from build123d import *

# Parameters (mm, degrees)
SKETCH_1_W              = 48
SKETCH_1_H              = 20
EXTRUDE_1_DEPTH         = 30
SKETCH_2_W              = 14
SKETCH_2_H              = 30
CUT_EXTRUDE_1_DEPTH     = 7
EXTRUDE_2_DEPTH         = 48
CUT_EXTRUDE_2_DEPTH     = 14
CUT_EXTRUDE_3_DEPTH     = 14
CUT_EXTRUDE_4_DEPTH     = 65.456478054
SKETCH_13_R             = 4
CUT_EXTRUDE_5_DEPTH     = 53.52066051
SKETCH_14_R             = 4
CUT_EXTRUDE_6_DEPTH     = 53.52066051
FILLET_1_R              = 7
EXTRUDE_3_DEPTH         = 3
EXTRUDE_5_DEPTH         = 1
SKETCH_20_R             = 7.5
CUT_EXTRUDE_8_DEPTH     = 53.520660579
BOSS_EXTRUDE1_DEPTH     = 25
CUT_EXTRUDE1_DEPTH      = 80.244164279
CUT_EXTRUDE1_DEPTH_BACK = 80.244164279


with BuildPart() as part:
    # Эскиз1 → Бобышка-Вытянуть1 (new body)
    with BuildSketch(Plane(origin=(0, 0, 0), x_dir=(1, 0, 0), z_dir=(0, 1, 0))):
        Rectangle(SKETCH_1_W, SKETCH_1_H)
    extrude(amount=EXTRUDE_1_DEPTH)

    # Эскиз2 → Вырез-Вытянуть1 (cut)
    with BuildSketch(Plane.XY.offset(10)):
        with Locations((0, 15)):
            Rectangle(SKETCH_2_W, SKETCH_2_H)
    extrude(amount=-CUT_EXTRUDE_1_DEPTH, mode=Mode.SUBTRACT)

    # Эскиз7 → Бобышка-Вытянуть2 (add)
    with BuildSketch(Plane(origin=(24, 0, 0), x_dir=(0, 0, -1), z_dir=(1, 0, 0))):
        Polygon((10, 0), (27.320508076, -10), (45.810889132, 22.026279442), (32, 30), (10, 30), align=None)
    extrude(amount=-EXTRUDE_2_DEPTH)

    # Эскиз8 → Вырез-Вытянуть2 (cut)
    with BuildSketch(Plane(origin=(24, 0, 0), x_dir=(0, 0, -1), z_dir=(1, 0, 0))):
        Polygon((10, 0), (10, 30), (32, 30), (45.810889132, 22.026279442), (27.320508076, -10), align=None)
    extrude(amount=-CUT_EXTRUDE_2_DEPTH, mode=Mode.SUBTRACT)

    # Эскиз9 → Вырез-Вытянуть3 (cut)
    with BuildSketch(Plane.ZY.offset(24)):
        Polygon((-10, 0), (-10, 30), (-32, 30), (-45.810889132, 22.026279442), (-27.320508076, -10), align=None)
    extrude(amount=-CUT_EXTRUDE_3_DEPTH, mode=Mode.SUBTRACT)

    # Эскиз11 → Вырез-Вытянуть4 (cut, through all)
    with BuildSketch(Plane.ZY.offset(10)):
        Polygon((-17.221869062, 5.518829477), (-27.321869062, 23.012542633), (-36.15532818, 17.912542633), (-26.05532818, 0.418829477), align=None)
    extrude(amount=-CUT_EXTRUDE_4_DEPTH, mode=Mode.SUBTRACT)

    # Эскиз13 → Вырез-Вытянуть5 (cut, through all)
    with BuildSketch(Plane(origin=(0, 0, -10), x_dir=(-1, 0, 0), z_dir=(0, 0, -1))):
        with Locations((17, 15)):
            Circle(SKETCH_13_R)
    extrude(amount=-CUT_EXTRUDE_5_DEPTH, mode=Mode.SUBTRACT)

    # Эскиз14 → Вырез-Вытянуть6 (cut, through all)
    with BuildSketch(Plane(origin=(0, 0, -10), x_dir=(-1, 0, 0), z_dir=(0, 0, -1))):
        with Locations((-17, 15)):
            Circle(SKETCH_14_R)
    extrude(amount=-CUT_EXTRUDE_6_DEPTH, mode=Mode.SUBTRACT)

    # Скругление1
    fillet_1_edges = [part.edges().sort_by_distance(p)[0] for p in [
        (-7, 15, 3),
        (7, 15, 3),
    ]]
    fillet(fillet_1_edges, radius=FILLET_1_R - 0.0001)  # a hair under: the kernel refuses the full size

    # Эскиз16 → Бобышка-Вытянуть3 (add)
    with BuildSketch(Plane(origin=(10, 0, 0), x_dir=(0, 0, -1), z_dir=(1, 0, 0))):
        Polygon((27.321869062, 23.012542633), (17.221869062, 5.518829477), (26.05532818, 0.418829477), (36.15532818, 17.912542633), align=None)
    extrude(amount=-EXTRUDE_3_DEPTH)

    # Эскиз18 → Бобышка-Вытянуть5 (add)
    with BuildSketch(Plane(origin=(0, -14.330127019, -24.820508076), x_dir=(-1, 0, 0), z_dir=(0, -0.49999999999998845, -0.8660254037844453))):
        with BuildLine():
            Line((3.076923077, 23.490381057), (3.076923077, 15.490381057))
            Line((3.076923077, 15.490381057), (-0.394230769, 15.490381057))
            add(Edge.make_bspline(
                [(-0.394230769, 15.490381057), (-0.475966203, 15.49101845), (-0.634155568, 15.49225205), (-0.863556464, 15.501067061), (-1.077173272, 15.519794557), (-1.276352297, 15.540710881), (-1.460752713, 15.571594241), (-1.630462401, 15.607825992), (-1.784830485, 15.650647709), (-1.925031539, 15.701264755), (-2.055118116, 15.758511595), (-2.175664232, 15.829183977), (-2.291845901, 15.906492451), (-2.399031866, 15.998074814), (-2.502049745, 16.096470161), (-2.596586483, 16.206601733), (-2.685439891, 16.325713037), (-2.793473896, 16.498197991), (-2.906939016, 16.729401784), (-3.004668447, 17.02314385), (-3.06681146, 17.330727068), (-3.073519576, 17.5408315), (-3.076923077, 17.647432339)],
                knots=[0, 0, 0, 0, 1.242075696, 2.40389213, 3.487198984, 4.500157661, 5.446319301, 6.326791195, 7.136300648, 7.878370406, 8.590488565, 9.292260633, 9.999224673, 10.708050372, 11.431369221, 12.162165018, 12.910600795, 13.687589445, 15.252257874, 16.810406251, 18.381693487, 20, 20, 20, 20], degree=3))
            add(Edge.make_bspline(
                [(-3.076923077, 17.647432339), (-3.075357604, 17.715865612), (-3.072265688, 17.851026019), (-3.048581646, 18.049748215), (-3.005726368, 18.239618444), (-2.950775925, 18.42230348), (-2.87555432, 18.595200652), (-2.788453183, 18.761894703), (-2.680395045, 18.917607923), (-2.559742342, 19.067544403), (-2.419445088, 19.204937793), (-2.263386964, 19.331922341), (-2.086876234, 19.440896432), (-1.89570213, 19.542168691), (-1.684937787, 19.625339579), (-1.457761732, 19.698574242), (-1.21241575, 19.755040234), (-1.042362796, 19.783482773), (-0.955128205, 19.798073364)],
                knots=[0, 0, 0, 0, 0.982645791, 1.940792824, 2.867691729, 3.775150443, 4.675643875, 5.571354211, 6.471357401, 7.392684514, 8.331098131, 9.285922955, 10.275520706, 11.304845665, 12.388884831, 13.524255008, 14.729980297, 16, 16, 16, 16], degree=3))
            add(Edge.make_bspline(
                [(-0.955128205, 19.798073364), (-1.019738399, 19.830278555), (-1.14226585, 19.891352818), (-1.308999482, 19.992404668), (-1.455065559, 20.087536339), (-1.53803712, 20.158871679), (-1.576923077, 20.192304134)],
                knots=[0, 0, 0, 0, 1.172551213, 2.223638478, 3.167479604, 4, 4, 4, 4], degree=3))
            add(Edge.make_bspline(
                [(-1.576923077, 20.192304134), (-1.652624383, 20.266285408), (-1.807875296, 20.418008818), (-2.019735444, 20.678834883), (-2.229368535, 20.965668904), (-2.355227865, 21.174690137), (-2.419871795, 21.282047723)],
                knots=[0, 0, 0, 0, 0.918170575, 1.883016652, 2.912673989, 4, 4, 4, 4], degree=3))
            Line((-2.419871795, 21.282047723), (-3.732371795, 23.490381057))
            Line((-3.732371795, 23.490381057), (-2.439102564, 23.490381057))
            Line((-2.439102564, 23.490381057), (-1.442307692, 21.801278493))
            add(Edge.make_bspline(
                [(-1.442307692, 21.801278493), (-1.406465761, 21.74201577), (-1.337009983, 21.627174345), (-1.236719552, 21.459429826), (-1.138255761, 21.30508177), (-1.047376022, 21.15932531), (-0.958316878, 21.02600434), (-0.878481314, 20.900073272), (-0.798305584, 20.788666158), (-0.706246053, 20.654823189), (-0.593818414, 20.510114732), (-0.462623309, 20.361457059), (-0.34199814, 20.238315643), (-0.18956943, 20.120822362), (-3.2323e-05, 20.013245791), (0.159774488, 19.962214344), (0.237179487, 19.937496441)],
                knots=[0, 0, 0, 0, 1.130591283, 2.190900266, 3.190104209, 4.119071823, 4.994606968, 5.807262858, 6.55236009, 7.234593472, 8.459046683, 9.540234366, 10.471327768, 11.266723835, 12.676093724, 14, 14, 14, 14], degree=3))
            add(Edge.make_bspline(
                [(0.237179487, 19.937496441), (0.269697183, 19.931632396), (0.343936058, 19.918244603), (0.469993483, 19.909501015), (0.622727518, 19.900220866), (0.733416476, 19.900491258), (0.793269231, 19.900637467)],
                knots=[0, 0, 0, 0, 0.709978628, 1.620902492, 2.713552433, 4, 4, 4, 4], degree=3))
            Line((0.793269231, 19.900637467), (1.948717949, 19.900637467))
            Line((1.948717949, 19.900637467), (1.948717949, 23.490381057))
            Line((1.948717949, 23.490381057), (3.076923077, 23.490381057))
        make_face()
        with BuildLine():
            Line((1.948717949, 18.977560544), (-0.193910256, 18.977560544))
            add(Edge.make_bspline(
                [(-0.193910256, 18.977560544), (-0.301354607, 18.97589409), (-0.502211742, 18.972778811), (-0.783007271, 18.945769758), (-1.023200158, 18.903550736), (-1.225858519, 18.839427155), (-1.396173113, 18.753553027), (-1.54378517, 18.648537277), (-1.667901131, 18.51825252), (-1.769975791, 18.368861713), (-1.849770319, 18.206056724), (-1.90552669, 18.03374763), (-1.942959563, 17.855238544), (-1.946787014, 17.733092852), (-1.948717949, 17.6714708)],
                knots=[0, 0, 0, 0, 1.546056516, 2.890207646, 4.055830773, 5.050253158, 5.937355789, 6.790906573, 7.644595853, 8.512568064, 9.38593768, 10.244184789, 11.114197691, 12, 12, 12, 12], degree=3))
            add(Edge.make_bspline(
                [(-1.948717949, 17.6714708), (-1.947235583, 17.626563151), (-1.944332064, 17.538602257), (-1.928948857, 17.409542216), (-1.89968097, 17.287236957), (-1.859266003, 17.17080484), (-1.808094758, 17.059993077), (-1.745213393, 16.955237495), (-1.670946372, 16.857073145), (-1.585753391, 16.765016757), (-1.487970747, 16.681241729), (-1.376270424, 16.608965458), (-1.251544399, 16.547545272), (-1.113644587, 16.498798364), (-0.963006292, 16.459808698), (-0.798771701, 16.43387015), (-0.621691971, 16.415101097), (-0.498985984, 16.414015918), (-0.435897436, 16.41345798)],
                knots=[0, 0, 0, 0, 0.965235723, 1.89061323, 2.787065514, 3.661873922, 4.534873316, 5.404925039, 6.281839248, 7.175200054, 8.095223355, 9.040740021, 10.02630299, 11.075573487, 12.177989335, 13.364883635, 14.645170704, 16, 16, 16, 16], degree=3))
            Line((-0.435897436, 16.41345798), (1.948717949, 16.41345798))
            Line((1.948717949, 16.41345798), (1.948717949, 18.977560544))
        make_face(mode=Mode.SUBTRACT)
    extrude(amount=EXTRUDE_5_DEPTH)

    # Эскиз20 → Вырез-Вытянуть8 (cut, through all)
    with BuildSketch(Plane(origin=(0, 0, -10), x_dir=(-1, 0, 0), z_dir=(0, 0, -1))):
        with Locations((-17, 15)):
            Circle(SKETCH_20_R)
        with Locations((17, 15)):
            Circle(SKETCH_20_R)
    extrude(amount=CUT_EXTRUDE_8_DEPTH, mode=Mode.SUBTRACT)

    # Sketch3 → Boss-Extrude1 (add)
    with BuildSketch(Plane(origin=(0, 30, 0), x_dir=(1, 0, 0), z_dir=(0, 1, 0))):
        with BuildLine():
            Line((7, -10), (24, -10))
            Line((24, -10), (24, 10))
            Line((24, 10), (10, 10))
            Line((10, 10), (10, 32))
            Line((10, 32), (-10, 32))
            Line((-10, 32), (-10, 10))
            Line((-10, 10), (-24, 10))
            Line((-24, 10), (-24, -10))
            Line((-24, -10), (-7, -10))
            ThreePointArc((-7, -10), (0, -3), (7, -10))
        make_face()
    extrude(amount=BOSS_EXTRUDE1_DEPTH)

    # Sketch4 → Cut-Extrude1 (cut, two sides: drawn at the far end of the back side and taken through both)
    with BuildSketch(Plane.ZY.offset(10).offset(-CUT_EXTRUDE1_DEPTH_BACK)):
        Polygon((-251.050138586, -96.468656479), (-45.810889132, 22.026279442), (35.63071017, 69.046608722), (240.869959624, 187.541544642), (3.880087783, 598.020043549), (-488.040010426, 314.009842428), align=None)
    extrude(amount=CUT_EXTRUDE1_DEPTH + CUT_EXTRUDE1_DEPTH_BACK, mode=Mode.SUBTRACT)


solid = part.part
Check sheet for the modelled part. Datum: model origin and axes. Units: mm. A direction names the side the tool comes from. Round coordinates to 2 decimals unless told otherwise and drop trailing zeros. Order: outer loops, then holes, each group sorted by start corner. A loop starts at its lowest first (then second) coordinate and runs counter-clockwise, first axis right, second up.
Q1. Set-up check for faces 1 (the face through (-1.619, 20.498, -31.677)), 2 (the face through (-1.949, 4, -36)), 3 (the face through (-10, 1, -22)): record each of +Z, -Z, +X, -X, +Y, -Y from which the full face is reachable in a straight line by a thin tool's end or side.
Filled sheet:
face 1: -X
face 2: -Z
face 3: -Z, -X, +Y, -Y
Q2. Cross-section at B-B, the plane y = 13.5. Give the number of separate pieces and of enclosed holes in the cut face, plus the area to 4 significant figures.
Filled sheet:
separate pieces: 3
enclosed holes: 0
area: 986.5 mm2
Q3. Scan lines: L1, parallel to X at y = 16, z = 2; L2, parallel to X at y = 8.5, z = -36; L3, parallel to Z at x = 0.5, y = 22.5. Record each from-to range of solid material in increasing order.
Filled sheet:
L1: x = -24 to -20.87, -13.13 to 13.13, 20.87 to 24
L2: x = -10 to 10
L3: z = -44.99 to -28.21, -27.03 to 3.02
Q4. Cross-section at A-A, the plane x = 17. Enter the section's corners in (y, z).
Filled sheet:
outline: (0, -10) - (11, -10) - (11, 10) - (0, 10) - close; (19, -10) - (42.7, -10) - (54.25, 10) - (19, 10) - close
Q5. Draft check along X on faces 4 (the face through (9.5, 15, -26.4)), 5 (the face through (-4.9, 15.2, 5)), 6 (the face through (-1.62, 14.14, -22.2)), 7 (the face through (-9.5, 15, -17)). Enter one of: pulls with the +X half, pulls with the -X half, needs draft (parallel to the pull), parting line crosses it, or undercut.
Filled sheet:
face 4: pulls with the +X half
face 5: undercut
face 6: needs draft
face 7: pulls with the -X half
Q6. Cross-section at D-D, the plane z = -3. Enter the section's corners in (x, y).
Filled sheet:
outline: (-24, 0) - (24, 0) - (24, 46.74) - (-24, 46.74) - close; hole circle Ø8 at (-17, 15); hole circle Ø8 at (17, 15)
Q7. Depth check by flat-ended pin: P1, Ø2, axis at y = 4, z = -36, coming from the +X side; P2, Ø3, axis at x = -9.5, z = -6, coming from the -Y side; P3, Ø7, axis at x = 15, y = 15.5, coming from the -Z side; P4, Ø3, axis at y = -1, z = -8.5, coming from the -X side. Enter the tip coordinate at first touch or a pass-through.
Filled sheet:
P1: stops at x = 10
P2: stops at y = 0
P3: stops at z = -10
P4: stops at x = -24
